Job drawing, mm, ordinate dimensions from the low corner. One solid piece. A direction names the side the tool comes from. Give positions to 0.01 mm unless a question says otherwise; leave off trailing zeros. Loops run counter-clockwise (first coordinate to the right, second up) from the corner with the lowest first, then second, coordinate; pieces in that order, holes last.
Item 1: Probe probe 1 along Z at (x, y) = (9.5, 5); probe 2 along X at (y, z) = (17.5, 34.5). List the from-to ranges inside material, lowest first.
Item 2: Mould opens along Z. For the marked faces 3, 4 and 5 say: released by +Z, released by -Z, zero draft, split by the parting line, or undercut.
Item 3: Saw through at A-A on z = 35.5. Give the cut face in (x, y), plus the area to 3 significant figures.
Item 4: Which spindle directions (+Z, -Z, +X, -X, +Y, -Y) get a long thin tool onto all of the face, cutting with end or side? Do the marked faces 1 and 2. Say none if no direction does.
Item 5: Saw through at C-C on y = 2.75. Give the cut face in (x, z), plus the area to 3 significant figures.
Item 6: Drop a flat-ended pin along its axis: P1, Ø5, axis at x = 58.5, z = 25, coming from the -Y side. Give the stop position or say it passes through.
Item 7: Saw through at B-B on x = 17. Give the cut face in (y, z).
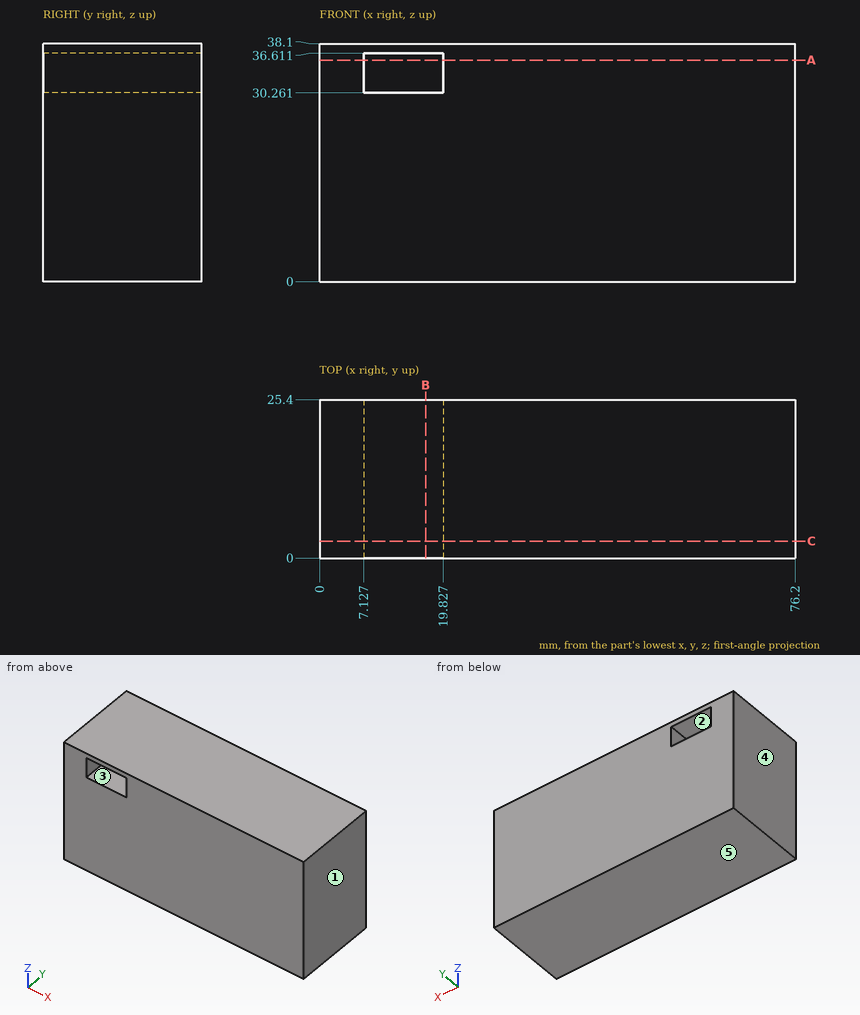
Results below:
1. probe 1: z = 0 to 30.26, 36.61 to 38.1
1. probe 2: x = 0 to 7.13, 19.83 to 76.2
2. face 3: undercut
2. face 4: zero draft
2. face 5: released by -Z
3. outline: (0, 0) - (7.13, 0) - (7.13, 25.4) - (0, 25.4) - close; (19.83, 0) - (76.2, 0) - (76.2, 25.4) - (19.83, 25.4) - close
3. area: 1,610 mm2
4. face 1: +Z, -Z, +X, +Y, -Y
4. face 2: +Y, -Y
5. outline: (0, 0) - (76.2, 0) - (76.2, 38.1) - (0, 38.1) - close; hole (7.13, 30.26) - (19.83, 30.26) - (19.83, 36.61) - (7.13, 36.61) - close
5. area: 2,820 mm2
6. P1: stops at y = 0
7. outline: (0, 0) - (25.4, 0) - (25.4, 30.26) - (0, 30.26) - close; (0, 36.61) - (25.4, 36.61) - (25.4, 38.1) - (0, 38.1) - close
